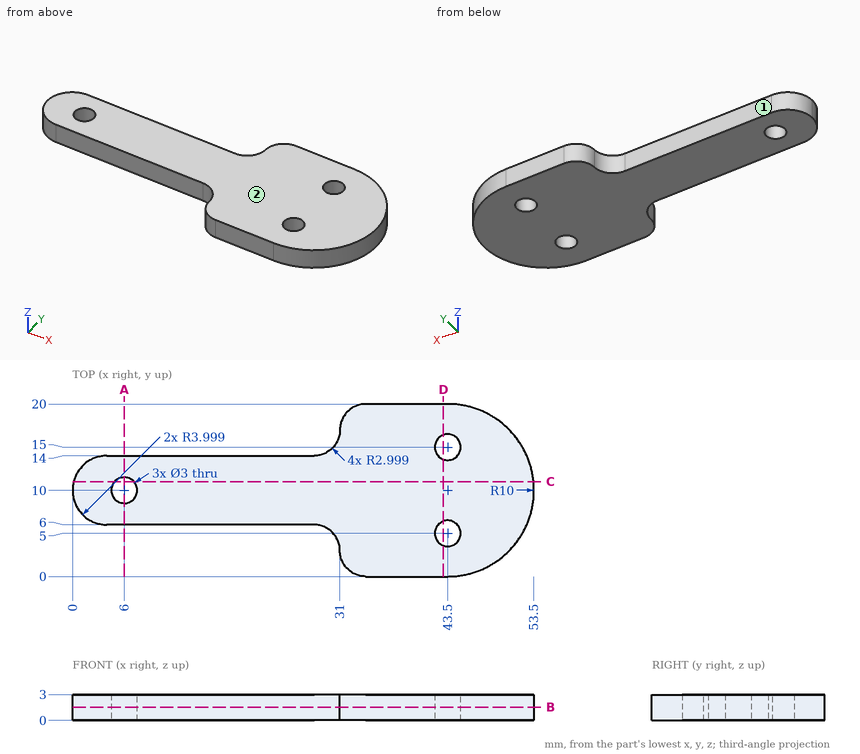
Verification items for this drawing (mm, ordinates from the low corner). A direction names the side the tool comes from. Coordinates: 2 decimals unless noted, no trailing zeros. Write each loop counter-clockwise with the first axis right and the second up, starting at its lowest first coordinate (ties: lowest second). Pieces come first, ordered by that corner, then holes. Notation, with made-up numbers: M -30.75,-15.5 L 17.25,-15.5 A15 ccw 17.25,5.5 Z; hole C 36.5,84 d11. An arc over 180 degrees is marked long. Use one line per item in the form item = value. Start each with the question number.
1) Thickness scan on probe 1 along Y at (x, z) = (43.5, 0.75); probe 2 along Y at (x, z) = (6, 1.3); probe 3 along Y at (x, z) = (8, 0.65). Record the ranges inside material, lowest first. Write a range as from..to.
2) Go/stop test with flat-tipped pins: pin 1 Ø3.5 at (x, y) = (43.5, 15) entering from -Z; pin 2 Ø1.5 at (y, z) = (11.5, 0.5) entering from +X; pin 3 Ø5 at (x, y) = (12.5, 17.5) entering from -Z; pin 4 Ø0.9 at (x, z) = (11.5, 1) entering from -Y. Record where each tip stops, or that it passes through.
3) Section check A-A on x = 6. Enter the section's corners in (y, z).
4) Set-up check for the marked faces 1 and 2: record each of +Z, -Z, +X, -X, +Y, -Y from which the full face is reachable in a straight line by a thin tool's end or side.
5) Section check B-B on z = 1.55. State how many separate pieces and enclosed holes the cut face has, and give its area (3 significant figures).
6) Section check C-C on y = 11. Enter the section's corners in (x, z).
7) Section check D-D on x = 43. Enter the section's corners in (y, z) (1 decimal).
Responses:
q1.probe_1 = 0..3.5, 6.5..13.5, 16.5..20
q1.probe_2 = 6..8.5, 11.5..14
q1.probe_3 = 6..14
q2.pin_1 = 0
q2.pin_2 = 53.47
q2.pin_3 = through
q2.pin_4 = 6
q3.outline = M 6,0 L 8.5,0 L 8.5,3 L 6,3 Z; M 11.5,0 L 14,0 L 14,3 L 11.5,3 Z
q4.face_1 = +Z, -Z, -X, +Y
q4.face_2 = +Z, +X, -X, +Y, -Y
q5.separate_pieces = 1
q5.enclosed_holes = 3
q5.area = 627 mm2
q6.outline = M 0.13,0 L 4.88,0 L 4.88,3 L 0.13,3 Z; M 7.12,0 L 53.45,0 L 53.45,3 L 7.12,3 Z
q7.outline = M 0,0 L 3.6,0 L 3.6,3 L 0,3 Z; M 6.4,0 L 13.6,0 L 13.6,3 L 6.4,3 Z; M 16.4,0 L 20,0 L 20,3 L 16.4,3 Z
